```python
from build123d import *

# Parameters (mm, degrees)
F2_R     = 15
F3_DEPTH = 50


with BuildPart() as f1:
    # F0 (on Right) → F1 (revolve)
    with BuildSketch(Plane.YZ):
        Polygon((15, 15), (0, 0), (-15, 15), (-25, 15), (-25, -45), (25, -45), (25, 15), align=None)
    revolve(axis=Axis((0, 0, -45), (0, 1, 0)))

    # F2 (on face) → F3 (cut)
    with BuildSketch(Plane.XZ.offset(25)):
        with Locations((0, -45)):
            Circle(F2_R)
    extrude(amount=-F3_DEPTH, mode=Mode.SUBTRACT)


solid = f1.part
```
Here's how the part is built. I have some questions about the finished solid (model axes, mm). A direction names the side the tool comes from. Coordinates: 2 decimals unless noted, no trailing zeros. Loops run counter-clockwise (first coordinate to the right, second up) from the corner with the lowest first, then second, coordinate; pieces in that order, holes last. Notation, with made-up numbers: (83, 84.5) -> (88, 84.5) arc R14 cw to (88, 88.5) -> close; hole circle Ø1 at (9, 26.5). An arc over 180 degrees is marked (long way). Return JSON: item names as keys, results as strings.
1) For faces 1 (the face through (13.7, 0.7, -1.4)), 2 (the face through (2.64, 19.93, -104.94)), which set-ups out of +Z, -Z, +X, -X, +Y, -Y let a thin tool reach every point of the face, with its end or its side?
Results below:
{"face 1": "none", "face 2": "+Y, -Y"}
2) I need wall thicknesses on line 1 (Z direction, x = -2, y = -19); line 2 (Z direction, x = 2, y = 3.5); line 3 (X direction, y = 15, z = -36.5). Which ranges of each line are inside material? Lowest first, please. Write a range as from..to.
Results below:
{"line 1": "-104.97..-59.87, -30.13..14.97", "line 2": "-93.46..-59.87, -30.13..3.46", "line 3": "-59.39..-12.36, 12.36..59.39"}
3) If we section it at C-C, the plane y = 9: Write out the boundary of the cut face in (x, z), then the cut area to 3 significant figures.
Results below:
{"outline": "circle Ø108 at (0, -45); hole circle Ø30 at (0, -45)", "area": "8,450 mm²"}
4) Will these pins go through, and if not, where does the flat tip stop? pin 1 (4 mm diameter, centred on x = -3, y = 7, fed in from +Z); pin 2 (1 mm diameter, centred on x = 14.5, y = 13.5, fed in from -Z); pin 3 (3 mm diameter, centred on x = 38.5, y = 15, fed in from +Z); pin 4 (18 mm diameter, centred on x = 0, z = -45, fed in from +Y).
Results below:
{"pin 1": "z = 8.92", "pin 2": "z = -102.21", "pin 3": "z = 2.23", "pin 4": "through"}
5) If we section it at D-D, the plane y = -10.5: Write out the boundary of the cut face in (x, z), then the cut area to 3 significant figures.
Results below:
{"outline": "circle Ø111 at (0, -45); hole circle Ø30 at (0, -45)", "area": "8,970 mm²"}
6) If we section it at A-A, the plane x = 0: Write out the boundary of the cut face in (y, z).
Results below:
{"outline": "(-25, -105) -> (-15, -105) -> (0, -90) -> (15, -105) -> (25, -105) -> (25, -60) -> (-25, -60) -> close; (-25, -30) -> (25, -30) -> (25, 15) -> (15, 15) -> (0, 0) -> (-15, 15) -> (-25, 15) -> close"}
7) If we section it at B-B, the plane z = -45: Write out the boundary of the cut face in (x, y).
Results below:
{"outline": "(-60, -25) -> (-15, -25) -> (-15, 25) -> (-60, 25) -> (-60, 15) -> (-45, 0) -> (-60, -15) -> close; (15, -25) -> (60, -25) -> (60, -15) -> (45, 0) -> (60, 15) -> (60, 25) -> (15, 25) -> close"}
8) Thinking about a two-plate mould opening in X: for faces 3 (the face through (-1.953, -0.35, -30.128)), 4 (the face through (2.64, -20.07, -104.94)), 5 (the face through (-12, -25, -33)), which applies, +X half, -X half, draft (parallel to the pull), parting line (faces both ways), or undercut?
Results below:
{"face 3": "undercut", "face 4": "parting line", "face 5": "draft"}
